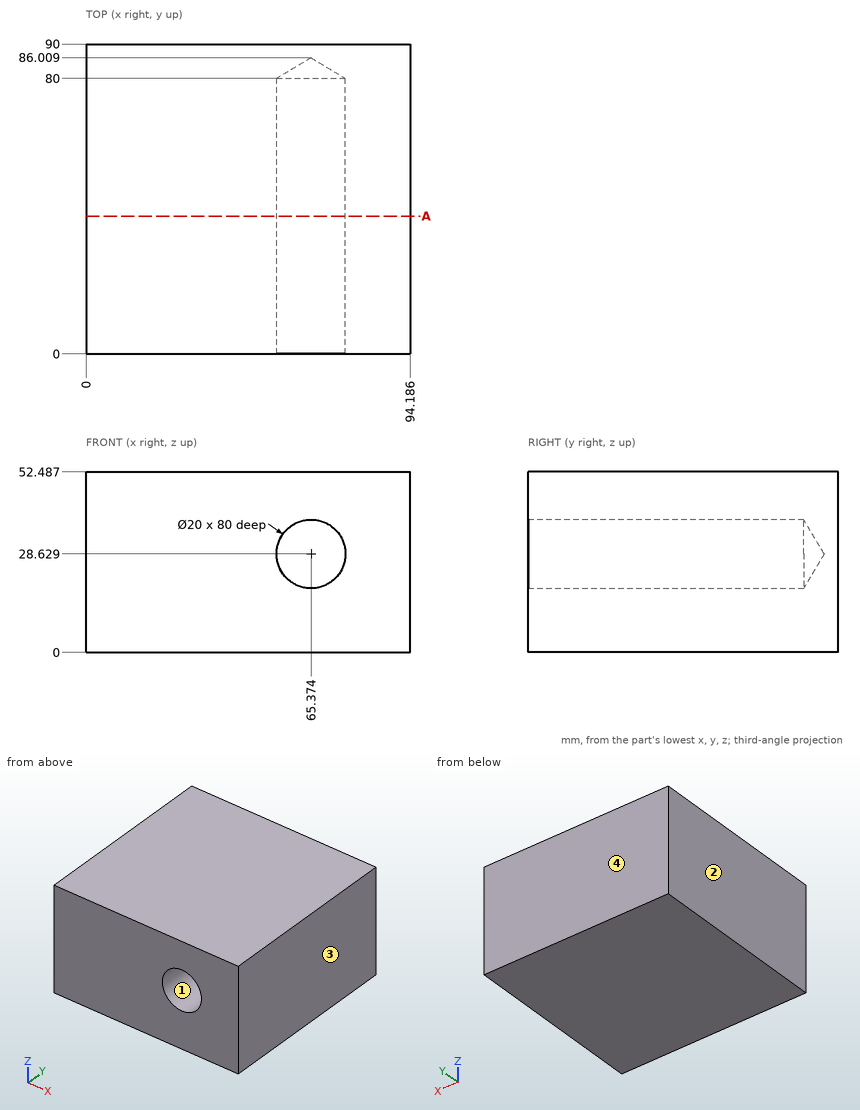
Here's the drawing with two shaded views (mm, measured from the low corner). I have some questions. Round coordinates to 2 decimals unless told otherwise and drop trailing zeros. Write each loop counter-clockwise with the first axis right and the second up, starting at its lowest first coordinate (ties: lowest second). Pieces come first, ordered by that corner, then holes. Notation, with made-up numbers: M 28.5,-39.75 L 87.5,-39.75 A28 ccw 87.5,-4.75 Z; hole C -23,59.25 d9. An arc over 180 degrees is marked long. Use CSV: the item, a comma, the result in double quotes.
(1) I need wall thicknesses on line 1 along Z through (x, y) = (62.5, 42.5); line 2 along X through (y, z) = (14.5, 29.5) (1 decimal); line 3 along Z through (x, y) = (64, 45) (1 decimal). Which ranges of each line are inside material? Lowest first, please.
Check values:
line 1,"0 to 19.05, 38.21 to 52.49"
line 2,"0 to 55.4, 75.3 to 94.2"
line 3,"0 to 18.7, 38.5 to 52.5"
(2) Imagine slicing it at A-A (y = 40). Write out the boundary of the cut face in (x, z) (1 decimal), plus the area to 3 significant figures.
Check values:
outline,"M 0,0 L 94.2,0 L 94.2,52.5 L 0,52.5 Z; hole C 65.4,28.6 d20"
area,"4,630 mm^2"
(3) I'm going to push a flat-ended pin straight in: pin 1 (6 mm diameter, centred on x = 69, z = 29, fed in from -Y) (1 decimal). Where does the tip first touch, or does it pass through?
Check values:
pin 1,"y = 82"
(4) We'd pull the mould along X, two halves only. Please class the marked faces 1, 2, 3 and 4: +X half, -X half, draft (parallel to the pull), parting line (faces both ways), or undercut.
Check values:
face 1,"undercut"
face 2,"-X half"
face 3,"+X half"
face 4,"draft"
